Part model, mm, in its own coordinate system. A direction names the side the tool comes from. Coordinates: 2 decimals unless noted, no trailing zeros. Loops run counter-clockwise (first coordinate to the right, second up) from the corner with the lowest first, then second, coordinate; pieces in that order, holes last. Notation, with made-up numbers: (0.5, 78.5) - (18.5, 78.5) arc R21 cw to (18.5, 93.5) - close; hole circle Ø11 at (75.5, -17.75). An arc over 180 degrees is marked (long way). Answer as CSV lines item,"result".
from build123d import *

# Parameters (mm, degrees)
GRUNDK_RPER_DEPTH = 2
VERRUNDUNG1_R     = 0.3
VERRUNDUNG2_R     = 0.3


with BuildPart() as part:
    # Skizze1 → Grundkörper (new body)
    with BuildSketch(Plane.XY):
        Polygon((0, -3.75), (0, 3.75), (-3.5, 3.75), (-3.5, 7.5), (4.2, 7.5), (4.2, 2.5), (7.5, 2.5), (7.5, -2.5), (4.2, -2.5), (4.2, -7.5), (-3.5, -7.5), (-3.5, -3.75), align=None)
    extrude(amount=GRUNDK_RPER_DEPTH)

    # Verrundung1
    verrundung1_edges = [part.edges().sort_by_distance(p)[0] for p in [
        (4.2, 7.5, 1),
        (4.2, 2.5, 1),
        (7.5, 2.5, 1),
        (7.5, -2.5, 1),
        (4.2, -2.5, 1),
        (4.2, -7.5, 1),
        (-3.5, -7.5, 1),
        (-3.5, -3.75, 1),
        (0, -3.75, 1),
        (0, 3.75, 1),
        (-3.5, 3.75, 1),
        (-3.5, 7.5, 1),
    ]]
    fillet(verrundung1_edges, radius=VERRUNDUNG1_R)

    # Verrundung2
    verrundung2_edges = [part.edges().sort_by_distance(p)[0] for p in [
        (0.35, 7.5, 0),
        (4.2, 5, 0),
        (5.85, 2.5, 0),
        (7.5, 0, 0),
        (5.85, -2.5, 0),
        (4.2, -5, 0),
        (0.35, -7.5, 0),
        (-3.5, -5.625, 0),
        (-1.75, -3.75, 0),
        (0, 0, 0),
        (-1.75, 3.75, 0),
        (-3.5, 5.625, 0),
        (7.412132034, -2.412132034, 0),
        (4.112132034, -7.412132034, 0),
        (-3.412132034, -7.412132034, 0),
        (-3.412132034, -3.837867966, 0),
        (-3.412132034, 3.837867966, 0),
        (-3.412132034, 7.412132034, 0),
        (7.412132034, 2.412132034, 0),
        (4.112132034, 7.412132034, 0),
        (4.287867966, 2.587867966, 0),
        (-0.087867966, 3.662132034, 0),
        (-0.087867966, -3.662132034, 0),
        (4.287867966, -2.587867966, 0),
    ]]
    fillet(verrundung2_edges, radius=VERRUNDUNG2_R)


solid = part.part
Q1. Saw through at B-B (z = 1.35). Give the cut face in (x, y).
Results:
outline,"(-3.5, -7.2) arc R0.3 ccw to (-3.2, -7.5) - (3.9, -7.5) arc R0.3 ccw to (4.2, -7.2) - (4.2, -2.8) arc R0.3 cw to (4.5, -2.5) - (7.2, -2.5) arc R0.3 ccw to (7.5, -2.2) - (7.5, 2.2) arc R0.3 ccw to (7.2, 2.5) - (4.5, 2.5) arc R0.3 cw to (4.2, 2.8) - (4.2, 7.2) arc R0.3 ccw to (3.9, 7.5) - (-3.2, 7.5) arc R0.3 ccw to (-3.5, 7.2) - (-3.5, 4.05) arc R0.3 ccw to (-3.2, 3.75) - (-0.3, 3.75) arc R0.3 cw to (0, 3.45) - (0, -3.45) arc R0.3 cw to (-0.3, -3.75) - (-3.2, -3.75) arc R0.3 ccw to (-3.5, -4.05) - close"
Q2. Two-plate mould, pull along Y, no slides. Class faces 1 (the face through (-2, 3.75, 1)), 2 (the face through (6, -2.5, 1)), 3 (the face through (2, 0, 2)): released by +Y, released by -Y, zero draft, split by the parting line, or undercut.
Results:
face 1,"undercut"
face 2,"released by -Y"
face 3,"zero draft"
Q3. Saw through at A-A (x = -0.5). Give the cut face in (y, z), then the cut area to 3 significant figures.
Results:
outline,"(-7.5, 0.3) arc R0.3 ccw to (-7.2, 0) - (-4.05, 0) arc R0.3 ccw to (-3.75, 0.3) - (-3.75, 2) - (-7.5, 2) - close; (3.75, 0.3) arc R0.3 ccw to (4.05, 0) - (7.2, 0) arc R0.3 ccw to (7.5, 0.3) - (7.5, 2) - (3.75, 2) - close"
area,"14.9 mm^2"
Q4. Saw through at D-D (x = 6.25). Give the cut face in (y, z), then the cut area to 3 significant figures.
Results:
outline,"(-2.5, 0.3) arc R0.3 ccw to (-2.2, 0) - (2.2, 0) arc R0.3 ccw to (2.5, 0.3) - (2.5, 2) - (-2.5, 2) - close"
area,"9.96 mm^2"
Q5. Which spindle directions (+Z, -Z, +X, -X, +Y, -Y) get a long thin tool onto all of the face, cutting with end or side? Do faces 4 (the face through (0, 0, 1)), 5 (the face through (4.2, -5, 1)), 6 (the face through (6, 2.5, 1)). Say none if no direction does.
Results:
face 4,"+Z, -Z, -X"
face 5,"+Z, -Z, +X, -Y"
face 6,"+Z, -Z, +X, +Y"
Q6. Flat gauge pins, fed straight in: pin 1 (0.8 mm diameter, centred on y = -6, z = 1, fed in from +X); pin 2 (0.5 mm diameter, centred on x = 5.5, z = 1, fed in from -Y). Where does each tip first touch, or does it go through?
Results:
pin 1,"stops at x = 4.2"
pin 2,"stops at y = -2.5"
Q7. Saw through at C-C (y = 3.25). Give the cut face in (x, z).
Results:
outline,"(0, 0.3) arc R0.3 ccw to (0.3, 0) - (3.9, 0) arc R0.3 ccw to (4.2, 0.3) - (4.2, 2) - (0, 2) - close"
Q8. Wall check: L1, parallel to Y at x = -3, z = 1; L2, parallel to X at y = 2.75, z = 1.8; L3, parallel to X at y = 7, z = 0.45. Give the ranges that are in metal, low to high.
Results:
L1,"y = -7.5 to -3.75, 3.75 to 7.5"
L2,"x = 0 to 4.2"
L3,"x = -3.5 to 4.2"
